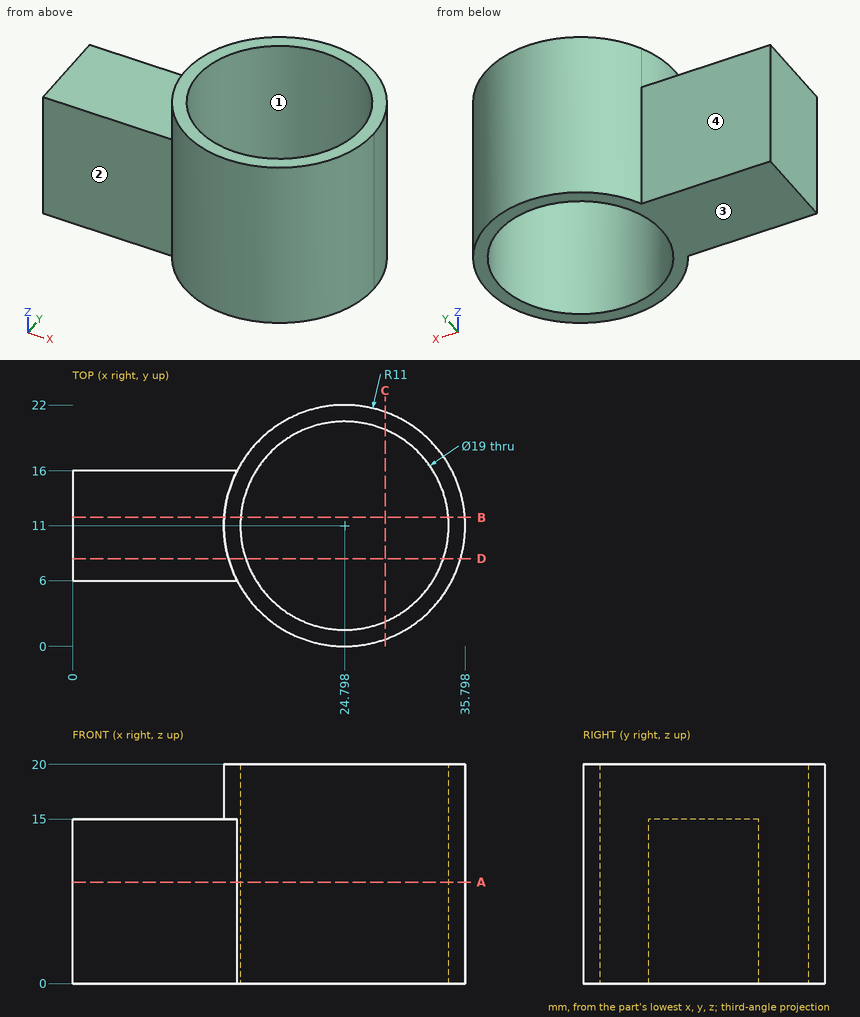
Here's the drawing with two shaded views (mm, measured from the low corner). I have some questions. Coordinates: 2 decimals unless noted, no trailing zeros. Loops run counter-clockwise (first coordinate to the right, second up) from the corner with the lowest first, then second, coordinate; pieces in that order, holes last. Notation, with made-up numbers: (43.25, -2) -> (80.25, -2) arc R17 cw to (80.25, 5) -> close; hole circle Ø4 at (74, 79). An arc over 180 degrees is marked (long way). Use one line per item in the form item = value. Start each with the question number.
(1) Please list where these lines run through material, in increasing order: line 1 along Y through (x, z) = (25, 17.75); line 2 along Y through (x, z) = (2.5, 14); line 3 along Y through (x, z) = (16.5, 9) (1 decimal).
(2) If we section it at C-C (x = 28.5): Please give me the cut outline in (y, z).
(3) Will these pins go through, and if not, where does the flat tip stop? pin 1 (5 mm diameter, centred on x = 9.5, y = 11, fed in from +Z); pin 2 (4 mm diameter, centred on y = 6.5, z = 14, fed in from +X); pin 3 (1.5 mm diameter, centred on y = 18.5, z = 3.5, fed in from -X).
(4) If we section it at B-B (y = 11.75): Please give me the cut outline in (x, z), then the cut area to 3 significant figures.
(5) If we section it at D-D (y = 8): Please give me the cut outline in (x, z) (3 decimals).
(6) We'd pull the mould along Y, two halves only. Please class the marked faces 1, 2, 3 and 4: pulls with the +Y half, pulls with the -Y half, needs draft (parallel to the pull), parting line crosses it, or undercut.
(7) If we section it at A-A (z = 9.25): Please give me the cut outline in (x, y).
Verdict:
q1.line_1 = 0 to 1.5, 20.5 to 22
q1.line_2 = 6 to 16
q1.line_3 = 3.8 to 6.4, 15.6 to 18.2
q2.outline = (0.64, 0) -> (2.25, 0) -> (2.25, 20) -> (0.64, 20) -> close; (19.75, 0) -> (21.36, 0) -> (21.36, 20) -> (19.75, 20) -> close
q3.pin_1 = 15
q3.pin_2 = 35.51
q3.pin_3 = 16.11
q4.outline = (0, 0) -> (15.33, 0) -> (15.33, 20) -> (13.82, 20) -> (13.82, 15) -> (0, 15) -> close; (34.27, 0) -> (35.77, 0) -> (35.77, 20) -> (34.27, 20) -> close
q4.area = 268 mm²
q5.outline = (0, 0) -> (15.784, 0) -> (15.784, 20) -> (14.215, 20) -> (14.215, 15) -> (0, 15) -> close; (33.812, 0) -> (35.381, 0) -> (35.381, 20) -> (33.812, 20) -> close
q6.face_1 = undercut
q6.face_2 = pulls with the -Y half
q6.face_3 = needs draft
q6.face_4 = pulls with the +Y half
q7.outline = (0, 6) -> (15, 6) arc R11 ccw (long way) to (15, 16) -> (0, 16) -> close; hole circle Ø19 at (24.8, 11)
